The listing builds one solid part. Answer for the finished solid, in the listing's coordinates (mm). A direction names the side the tool comes from. Give positions to 0.01 mm unless a question says otherwise; leave off trailing zeros. Order: outer loops, then holes, each group sorted by start corner. A loop starts at its lowest first (then second) coordinate and runs counter-clockwise, first axis right, second up.
```python
from build123d import *

# Parameters (mm, degrees)
SKETCH1_R           = 1.25
BOSS_EXTRUDE1_DEPTH = 2
CIRPATTERN1_COUNT   = 4
FILLET1_R           = 4
CUT_EXTRUDE1_DEPTH  = 8


with BuildPart() as part:
    # Sketch1 → Boss-Extrude1 (new body)
    with BuildSketch(Plane(origin=(0, 0, 0), x_dir=(1, 0, 0), z_dir=(0, 1, 0))):
        with BuildLine():
            Line((0, 4), (0, -4))
            Line((0, -4), (-8, -4))
            ThreePointArc((-8, -4), (-9.414213562, -3.414213562), (-10, -2))
            Line((-10, -2), (-10, 2))
            ThreePointArc((-10, 2), (-9.414213562, 3.414213562), (-8, 4))
            Line((-8, 4), (0, 4))
        make_face()
        with Locations((-5, 0)):
            Circle(SKETCH1_R, mode=Mode.SUBTRACT)
    boss_extrude1 = extrude(amount=BOSS_EXTRUDE1_DEPTH)

    # Sketch2 → Revolve1 (revolve)
    with BuildSketch(Plane.XY):
        Polygon((0, 2), (0, -2), (15, -12), (25, -12), (25, -8), (15, -8), align=None)
    revolve(axis=Axis((-9.784018472, -18, 0), (1, 0, 0)))

    # CirPattern1: Boss-Extrude1 ×4 about axis
    cirpattern1_axis = Axis((0, -18, 0), (1, 0, 0))
    for i in range(1, CIRPATTERN1_COUNT):
        add(boss_extrude1.rotate(cirpattern1_axis, i * 360 / CIRPATTERN1_COUNT))

    # Fillet1
    fillet1_edges = [part.edges().sort_by_distance(p)[0] for p in [
        (15, -28, 0),
    ]]
    fillet(fillet1_edges, radius=FILLET1_R)

    # Sketch3 → Cut-Extrude1 (cut)
    with BuildSketch(Plane(origin=(25, 0, 0), x_dir=(0, 0, -1), z_dir=(1, 0, 0))):
        Polygon((1, -12), (1, -11), (-1, -11), (-1, -12), (-1, -12.906953831), (1, -12.906953831), align=None)
    extrude(amount=-CUT_EXTRUDE1_DEPTH, mode=Mode.SUBTRACT)


solid = part.part
```
1) Straight lines are drawn through the part: probe 1 along Y at (x, z) = (-5, 19); probe 2 along Z at (x, y) = (-5, 1.3); probe 3 along Z at (x, y) = (22, -18). For each, find the intervals that lie inside material, in ascending order.
Geometry says:
probe 1: y = -22 to -19.25, -16.75 to -14
probe 2: z = -4 to -1.25, 1.25 to 4
probe 3: z = -10 to -6, 6 to 10
2) Find section C-C (x = 11.5). Write down the section's boundary in (y, z), then the cut area to 3 significant figures.
Geometry says:
outline: circle Ø24.67 at (-18, 0); hole circle Ø16.67 at (-18, 0)
area: 260 mm2
3) Find section A-A (x = -5). Count the separate pieces of the cut face and the enclosed holes in it, then the cut area to 3 significant figures.
Geometry says:
separate pieces: 8
enclosed holes: 0
area: 44.0 mm2
4) A tool of negligible diameter and unlimited length cuts with its end or side. For faces 1 (the flat face through (21.1, -11.5, 1)), 2 (the flat face through (-4, 1, -4)), 3 (the flat face through (-4, -37, 4)), from which of +Z, -Z, +X, -X, +Y, -Y can it reach the whole face along a straight path? Write none if from no direction.
Geometry says:
face 1: +X
face 2: -Z, -X, +Y, -Y
face 3: +Z, -X, +Y, -Y
5) For a pull along X with two mould halves and no side action, classify faces 4 (the flat face through (21.1, -11.5, -1)), 5 (the cylindrical face through (-5.27, -16.78, -18.99)), 6 (the conical face through (12.605, -25.589, 0.334)) as +X half, -X half, draft (parallel to the pull), parting line (faces both ways), or undercut.
Geometry says:
face 4: draft
face 5: undercut
face 6: -X half
6) Given P1, Ø2, axis at x = -5, y = -18, coming from the +Z side; P2, Ø2, axis at x = 8.5, z = -0.5, coming from the +Y side; P3, Ø0.9, axis at x = 19.5, y = -11.5, coming from the +Z side; P4, Ø6, axis at x = 18.5, y = -12.5, coming from the +Z side, each flat-ended and moving along its own axis, determine where each tip first touches the part or whether it passes through.
Geometry says:
P1: passes through
P2: stops at y = -3.01
P3: stops at z = 7.96
P4: stops at z = 9.68
7) Find section B-B (x = 20). Write down the section's boundary in (y, z), then the cut area to 3 significant figures.
Geometry says:
outline: circle Ø20 at (-18, 0); hole (-12.08, -1) - (-11, -1) - (-11, 1) - (-12.08, 1) arc R6 ccw (long way) to start
area: 199 mm2
